Geometry: see drawing. Coordinates: mm, zero at the bounding-box minimum. Coordinates: 2 decimals unless noted, no trailing zeros. Loops run counter-clockwise (first coordinate to the right, second up) from the corner with the lowest first, then second, coordinate; pieces in that order, holes last. Notation, with made-up numbers: (89.25, 18.25) - (138.25, 18.25) arc R32 ccw to (138.25, 56.25) - close; hole circle Ø7 at (84.25, 27.25). An arc over 180 degrees is marked (long way). Write item = value, one per line. Start each with the question number.
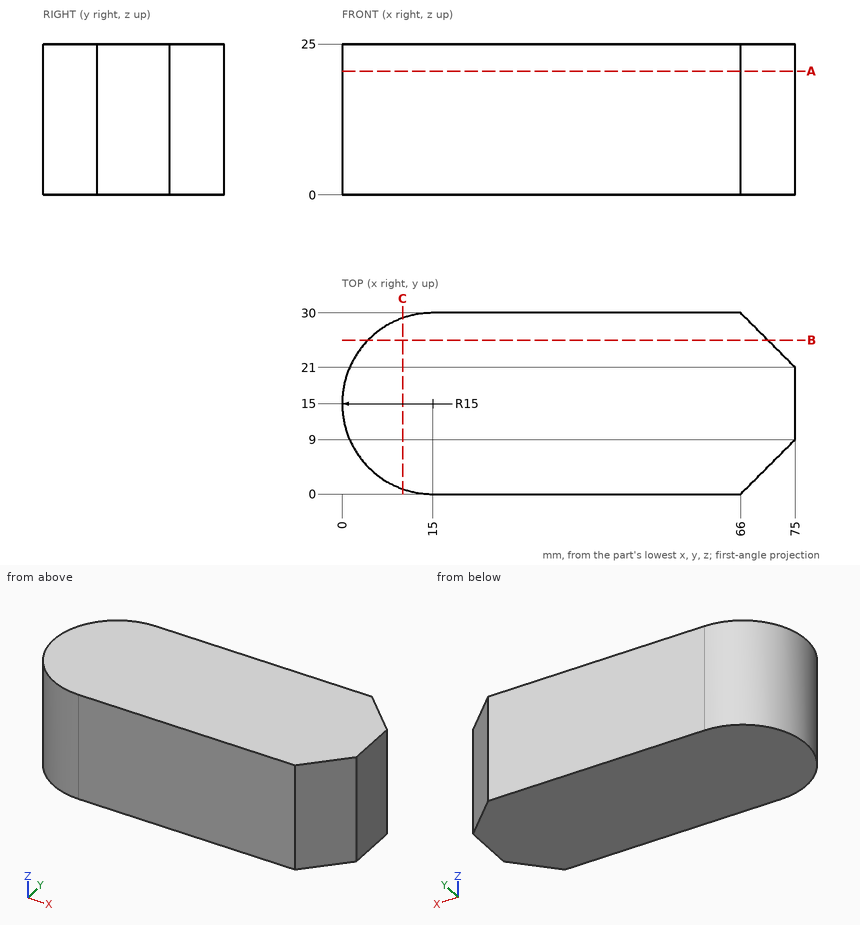
Item 1: Cut plane A-A (z = 20.5). Return the cut outline in (x, y).
Item 2: Cut plane C-C (x = 10). Return the cut outline in (y, z).
Item 3: First-contact query: pin 1 (8 mm diameter, centred on x = 9.5, y = 14.5, fed in from -Z); pin 2 (1.5 mm diameter, centred on y = 19, z = 7, fed in from -X); pin 3 (1.5 mm diameter, centred on y = 25.5, z = 12.5, fed in from +X); pin 4 (3 mm diameter, centred on y = 23, z = 22, fed in from -X). Flat tips, straight axial feed; report the tip coordinate or a pass-through.
Item 4: Cut plane B-B (y = 25.5). Return the cut outline in (x, z).
Item 5: Material intervals for L1, parallel to X at y = 5.75, z = 23.75; L2, parallel to X at y = 25, z = 8; L3, parallel to Y at x = 10, z = 9.75, sorted ascending. Write a range as [from, to].
Responses:
q1.outline = (15, 0) - (66, 0) - (75, 9) - (75, 21) - (66, 30) - (15, 30) arc R15 ccw to start
q2.outline = (0.86, 0) - (29.14, 0) - (29.14, 25) - (0.86, 25) - close
q3.pin_1 = 0
q3.pin_2 = 0.36
q3.pin_3 = 71.25
q3.pin_4 = 1.48
q4.outline = (4.29, 0) - (70.5, 0) - (70.5, 25) - (4.29, 25) - close
q5.L1 = [3.19, 71.75]
q5.L2 = [3.82, 71]
q5.L3 = [0.86, 29.14]
